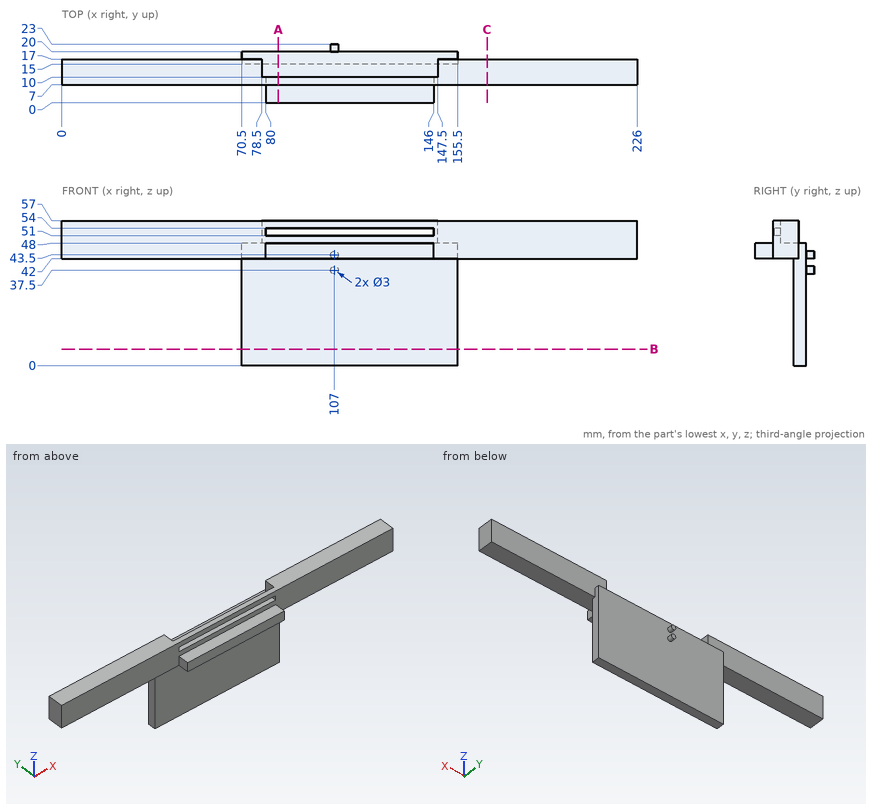
Input: dimensioned drawing with shaded views. Units: mm. Origin: part minimum x, y, z. Round coordinates to 2 decimals unless told otherwise and drop trailing zeros. Loops run counter-clockwise (first coordinate to the right, second up) from the corner with the lowest first, then second, coordinate; pieces in that order, holes last.
1) Pin query (flat end, axial travel): pin 1 (1.5 mm diameter, centred on y = 17.5, z = 15, fed in from -X); pin 2 (1.8 mm diameter, centred on y = 4, z = 44.5, fed in from -X); pin 3 (2.5 mm diameter, centred on x = 127, y = 8.5, fed in from -Z). Return the tip coordinate at first contact, or that it passes through.
Ans:
pin 1: stops at x = 70.5
pin 2: stops at x = 80
pin 3: stops at z = 42
2) Material intervals for line 1 (Z direction, x = 129, y = 9.75); line 2 (Z direction, x = 116.5, y = 18); line 3 (Y direction, x = 191, z = 48), sorted ascending.
Ans:
line 1: z = 42 to 51, 54 to 57
line 2: z = 0 to 48
line 3: y = 7 to 17
3) Section query A-A on x = 85. Return the cut outline in (y, z).
Ans:
outline: (0, 42) - (15, 42) - (15, 0) - (20, 0) - (20, 48) - (10, 48) - (10, 51) - (7, 51) - (7, 48) - (0, 48) - close; (7, 54) - (10, 54) - (10, 57) - (7, 57) - close
4) Section query C-C on x = 167. Return the cut outline in (y, z), plus the area to 3 significant figures.
Ans:
outline: (7, 42) - (17, 42) - (17, 57) - (7, 57) - close
area: 150 mm2
5) Section query B-B on z = 6.5. Return the cut outline in (x, y).
Ans:
outline: (70.5, 15) - (155.5, 15) - (155.5, 20) - (70.5, 20) - close
